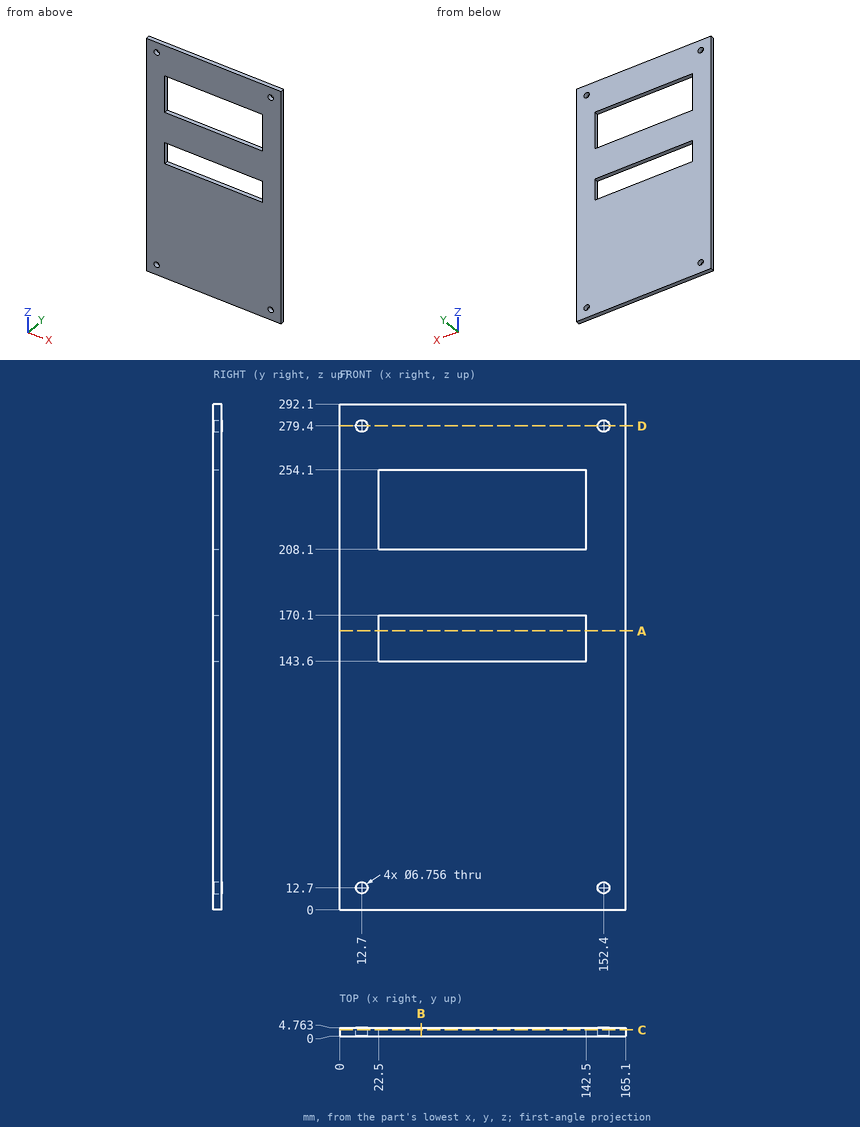
Part print with two shaded views. Sizes in mm from the minimum x, y, z corner. Coordinates: 2 decimals unless noted, no trailing zeros. Order: outer loops, then holes, each group sorted by start corner. A loop starts at its lowest first (then second) coordinate and runs counter-clockwise, first axis right, second up. Notation, with made-up numbers: (35, -35.75) - (63, -35.75) arc R15 ccw to (63, -17.75) - close; hole circle Ø11 at (18, 26.5). An arc over 180 degrees is marked (long way). Answer in a Markdown table with one row per item.
1. Slice it at A-A, the plane z = 161. List the corners of the cut face in (x, y), then the cut area to 3 significant figures.
Answer:
| item | result |
|---|---|
| outline | (0, 0) - (22.5, 0) - (22.5, 4.76) - (0, 4.76) - close; (142.5, 0) - (165.1, 0) - (165.1, 4.76) - (142.5, 4.76) - close |
| area | 215 mm² |
2. Slice it at B-B, the plane x = 47. List the corners of the cut face in (y, z).
Answer:
| item | result |
|---|---|
| outline | (0, 0) - (4.76, 0) - (4.76, 143.6) - (0, 143.6) - close; (0, 170.1) - (4.76, 170.1) - (4.76, 208.1) - (0, 208.1) - close; (0, 254.1) - (4.76, 254.1) - (4.76, 292.1) - (0, 292.1) - close |
3. Slice it at D-D, the plane z = 279.4. List the corners of the cut face in (x, y).
Answer:
| item | result |
|---|---|
| outline | (0, 0) - (9.32, 0) - (9.32, 4.76) - (0, 4.76) - close; (16.08, 0) - (149.02, 0) - (149.02, 4.76) - (16.08, 4.76) - close; (155.78, 0) - (165.1, 0) - (165.1, 4.76) - (155.78, 4.76) - close |
4. Drill centre lines: L1, parallel to Z at x = 60.5, y = 2.2; L2, parallel to Z at x = 152.4, y = 1.85; L3, parallel to X at y = 2.5, z = 279.4. Where is each one in solid material? Low to high. Write a range as from..to.
Answer:
| item | result |
|---|---|
| L1 | 0..143.6, 170.1..208.1, 254.1..292.1 |
| L2 | 0..9.32, 16.08..276.02, 282.78..292.1 |
| L3 | 0..9.32, 16.08..149.02, 155.78..165.1 |
5. Flat gauge pin, fed straight in: P1, Ø2.5, axis at x = 56.5, y = 2.5, coming from the -Z side. Where does the tip first touch, or does it go through?
Answer:
| item | result |
|---|---|
| P1 | z = 0 |
6. Slice it at C-C, the plane y = 3.5. List the corners of the cut face in (x, z).
Answer:
| item | result |
|---|---|
| outline | (0, 0) - (165.1, 0) - (165.1, 292.1) - (0, 292.1) - close; hole circle Ø6.76 at (12.7, 12.7); hole circle Ø6.76 at (12.7, 279.4); hole (22.5, 143.6) - (142.5, 143.6) - (142.5, 170.1) - (22.5, 170.1) - close; hole (22.5, 208.1) - (142.5, 208.1) - (142.5, 254.1) - (22.5, 254.1) - close; hole circle Ø6.76 at (152.4, 12.7); hole circle Ø6.76 at (152.4, 279.4) |
